Build history of the part. All positions in model axes, mm. Face numbers are marked on the shaded views. Round coordinates to 2 decimals unless told otherwise and drop trailing zeros. Write each loop counter-clockwise with the first axis right and the second up, starting at its lowest first coordinate (ties: lowest second). Pieces come first, ordered by that corner, then holes. Notation, with made-up numbers: M 37,-24 L 90,-24 A12 cw 90,-19 Z; hole C 59.25,-20.75 d6. An arc over 180 degrees is marked long. Use a Markdown table: item, result.
Autodesk Inventor part; units mm, degrees
ref_plane "YZ Plane" through (0, 0, 0) normal (1, 0, 0) x (0, 1, 0)
ref_plane "XZ Plane" through (0, 0, 0) normal (0, 1, 0) x (-1, 0, 0)
ref_plane "XY Plane" through (0, 0, 0) normal (0, 0, 1) x (1, 0, 0)
sketch "Skizze1" plane through (0, 0, 0) normal (0, 0, 1) x (1, 0, 0)
  line L0 (0, 70.8) -> (0, -11.8)
  line L1 (-25.8, 0) -> (4.3, 0)
  line L2 (-21.5, 0) -> (-21.5, 5)
  line L3 (-21.5, 5) -> (-5, 5)
  line L4 (-5, 5) -> (-5, 59)
  line L5 (-5, 59) -> (0, 59)
  line L6 (0, 59) -> (0, 0)
  line L7 (0, 0) -> (-21.5, 0)
  dimension "d0" = 16.5
  dimension "d1" = 5
  dimension "d2" = 5
  dimension "d3" = 54
extrude "Extrusion1" add sketch "Skizze1" along normal blind 70
sketch "Skizze2" plane through (-21.5, 5, 0) normal (0, 1, 0) x (1, 0, 0)
  line L0 (0, -70) -> (16.5, -70)
  line L1 (0, 0) -> (0, -70)
  point P0 (21.5, 0)
  point P1 (5, -62.5)
  point P2 (5, -27.5)
  dimension "d6" = 35
  dimension "d7" = 5
  dimension "d8" = 5
  dimension "d9" = 7.5
hole "Bohrung1" at (-16.5, 5, 62.5) at (-16.5, 5, 27.5) direction (0, -1, 0) diameter 4.2 end through all countersink diameter 9 countersink angle 90
sketch "Skizze3" plane through (-21.5, 5, 0) normal (0, 1, 0) x (1, 0, 0)
  circle A0 centre (5, -27.5) radius 4.5
  circle A1 centre (5, -62.5) radius 4.5
  line L0 (0, 0) -> (0, -70)
  line L1 (5, -62.5) -> (5, -27.5) construction
  circle A2 centre (5, -45) radius 4
  point P0 (21.5, 0)
  dimension "d18" = 17.5
  dimension "d19" = 8
extrude "Extrusion2" cut sketch "Skizze3" against normal up to surface (5 mm away) contours A2
sketch "Skizze4" plane through (0, 0, 0) normal (1, 0, 0) x (0, 0, -1)
  line L0 (-70, 59) -> (-70, 0)
  line L1 (0, 59) -> (-70, 59)
  circle A0 centre (-34, 39.5) radius 2.067
  circle A1 centre (-8, 39.5) radius 2.067
  point P0 (-54, 49.5)
  point P1 (-28, 49.5)
  dimension "d34" = 9.5
  dimension "d35" = 9.5
  dimension "d36" = 16
  dimension "d37" = 26
hole "Bohrung2" at (0, 49.5, 54) at (0, 49.5, 28) direction (-1, 0, 0) diameter 5.3 end through all countersink diameter 12 countersink angle 90
sketch "Skizze5" plane through (-5, 5, 0) normal (-1, 0, 0) x (0, 0, 1)
  line L0 (0, 54) -> (70, 54)
  line L1 (0, 54) -> (0, 0)
  circle A0 centre (10, 29.5) radius 6
  circle A1 centre (28, 44.5) radius 2.067
  circle A2 centre (54, 44.5) radius 2.067
  circle A3 centre (18.5, 60.5) radius 2.2
  line L2 (62, 72) -> (62, 35)
  line L3 (62, 72) -> (-5.5, 72)
  arc A4 (-28, 90.2303) -> (-5.5, 72) centre (-5.5, 95) ccw
  line L4 (-28, 15) -> (-28, 90.2303)
  line L5 (-28, 15) -> (-18, 15)
  line L6 (-18, 35) -> (-18, 15)
  line L7 (62, 35) -> (-18, 35)
  circle A5 centre (28, 44.5) radius 2.65
  circle A6 centre (54, 44.5) radius 2.65
  line L8 (70, 0) -> (70, 54)
  line L9 (0, 54) -> (70, 54)
  line L10 (0, 54) -> (0, 0)
  line L11 (0, 0) -> (70, 0)
  line L12 (32.75, 18) -> (32.75, 106)
  point P0 (0, -5)
  dimension "d38" = 24.5
  dimension "d39" = 12
  dimension "d40" = 10
extrude "Extrusion3" cut sketch "Skizze5" against normal blind 5 contours L7 A0 | A0 L7
sketch "Skizze7" plane through (0, 0, 0) normal (0, 0, -1) x (-1, 0, 0)
  line L0 (0, 28.5) -> (0, 40.5)
  line L1 (0, 28.5) -> (0, 40.5)
  line L2 (5, 40.5) -> (5, 28.5)
  line L3 (5, 28.5) -> (0, 28.5)
  line L4 (5, 40.5) -> (0, 40.5)
  point P0 (2.5, 34.5)
hole "Bohrung3" at (-2.5, 34.5, 0) direction (0, 0, 1) diameter 2.013 end up to surface
sketch "Skizze8" plane through (-5, 5, 0) normal (-1, 0, 0) x (0, 0, 1)
  line L0 (0, 0) -> (70, 0)
  line L1 (70, 54) -> (62, 54)
  line L2 (62, 54) -> (62, 0)
  line L3 (62, 0) -> (70, 0)
  line L4 (70, 0) -> (70, 54)
  point P0 (0, -5)
  dimension "d50" = 8
extrude "Extrusion4" cut sketch "Skizze8" against normal blind 5
equation "\"d2\" = d1"
properties part number "Motorhalter" material "Aluminum-6061"
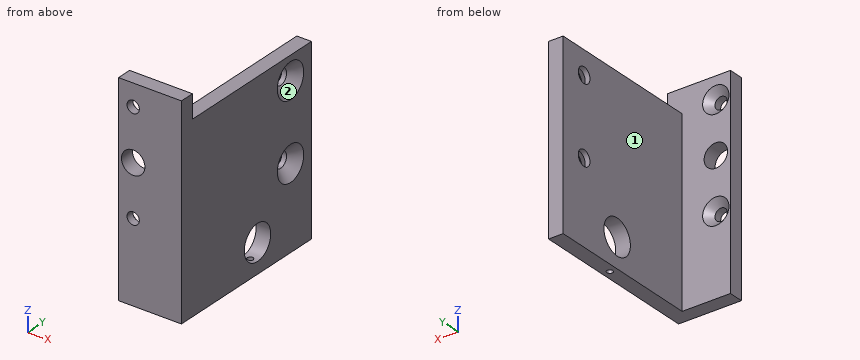
Q1. Drill centre lines: L1, parallel to Z at x = -16.5, y = 0.6; L2, parallel to Y at x = -3.8, z = 10; L3, parallel to X at y = 3.3, z = 45. Where is each one in solid material? Low to high.
Response values:
| item | result |
|---|---|
| L1 | z = 0 to 25.4, 29.6 to 41, 49 to 60.4, 64.6 to 70 |
| L2 | y = 0 to 28.5, 40.5 to 59 |
| L3 | x = -21.5 to -20.5, -12.5 to 0 |
Q2. Cut at A-A on x = -16.5. Give the cut face in (y, z).
Response values:
| item | result |
|---|---|
| outline | M 0,0 L 5,0 L 5,23 L 2.6,25.4 L 0,25.4 Z; M 0,29.6 L 2.6,29.6 L 5,32 L 5,41 L 0,41 Z; M 0,49 L 5,49 L 5,58 L 2.6,60.4 L 0,60.4 Z; M 0,64.6 L 2.6,64.6 L 5,67 L 5,70 L 0,70 Z |
Q3. Cut at D-D on y = 34.5. Give the cut face in (x, z).
Response values:
| item | result |
|---|---|
| outline | M -5,0 L -3.51,0 L -3.51,4 L -5,4 Z; M -5,16 L 0,16 L 0,62 L -5,62 Z; M -1.49,0 L 0,0 L 0,4 L -1.49,4 Z |
Q4. Drop flat-ended pins along their axis: P1, Ø7, axis at y = 49.5, z = 28, coming from the +X side; P2, Ø5.5, axis at x = -2.5, y = 27, coming from the +Z side; P3, Ø7, axis at y = 34.5, z = 10, coming from the +X side; P4, Ø6.5, axis at x = -8.5, z = 44, coming from the +Y side. Give the stop position or say it passes through.
Response values:
| item | result |
|---|---|
| P1 | stops at x = -2.5 |
| P2 | stops at z = 62 |
| P3 | passes through |
| P4 | stops at y = 5 |
Q5. Cut at B-B on y = 49.5. Give the cut face in (x, z), and give its area (3 significant figures).
Response values:
| item | result |
|---|---|
| outline | M -5,0 L 0,0 L 0,22 L -3.35,25.35 L -5,25.35 Z; M -5,30.65 L -3.35,30.65 L 0,34 L 0,48 L -3.35,51.35 L -5,51.35 Z; M -5,56.65 L -3.35,56.65 L 0,60 L 0,62 L -5,62 Z |
| area | 235 mm2 |
Q6. Cut at C-C on z = 10. Give the cut face in (x, y).
Response values:
| item | result |
|---|---|
| outline | M -21.5,0 L 0,0 L 0,28.5 L -5,28.5 L -5,5 L -21.5,5 Z; M -5,40.5 L 0,40.5 L 0,59 L -5,59 Z |
Q7. Two-plate mould, pull along Z, no slides. Class the marked faces 1 and 2: +Z half, -Z half, draft (parallel to the pull), parting line (faces both ways), or undercut.
Response values:
| item | result |
|---|---|
| face 1 | draft |
| face 2 | undercut |
